For this review, take the finished solid that the model builds, in its own axes (mm). Face numbers are marked on the shaded views. A direction names the side the tool comes from. Coordinates: 2 decimals unless noted, no trailing zeros. Order: outer loops, then holes, each group sorted by start corner. A loop starts at its lowest first (then second) coordinate and runs counter-clockwise, first axis right, second up. Notation, with made-up numbers: (88, -24.5) -> (125, -24.5) arc R15 ccw to (125, -1.5) -> close; hole circle Ø8 at (84.5, -37). An arc over 180 degrees is marked (long way). Write item = value, one per line. Start each with the question number.
1) Consider section C-C on z = -25. Give the boundary of the cut face in (x, y), and give its area (3 significant figures).
2) Insertion check: pin 1 Ø8 at (x, y) = (-24.5, 14) entering from +Z; pin 2 Ø1 at (y, z) = (8, -37.5) entering from +X; pin 3 Ø3 at (x, y) = (-27, 6.5) entering from -Z; pin 4 Ø3 at (x, y) = (-26, 5) entering from -Z. Each pin has a flat end and moves straight along its axis. Give the tip position at first contact, or say it passes through.
3) Wall thickness on probe 1 along Y at (x, z) = (-26, -28.7); probe 2 along X at (y, z) = (9, -33); probe 3 along Z at (x, y) = (-6, 5.5): over which ranges is each line inside the solid? List them lowest first. Write a range as [from, to].
4) Consider section A-A on x = -26. Give the boundary of the cut face in (y, z), and give its area (3 significant figures).
5) Machinability: for the marked faces 1, 2, 3 and 4, which of the approach directions +Z, -Z, +X, -X, +Y, -Y give a long, thin tool a straight path to every point of the face, cutting with its end or side? Answer none if there is none.
6) Consider section D-D on x = -6. Give the boundary of the cut face in (y, z), and give its area (3 significant figures).
7) Consider section B-B on y = 15. Give the boundary of the cut face in (x, z).
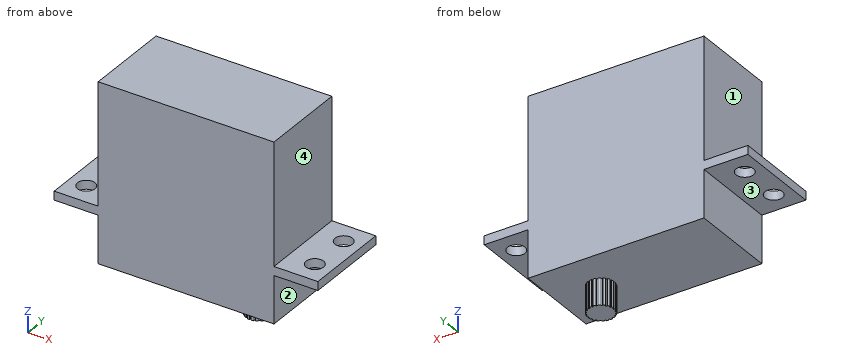
Autodesk Inventor part; units mm, degrees
ref_plane "YZ Plane" through (0, 0, 0) normal (1, 0, 0) x (0, 1, 0)
ref_plane "XZ Plane" through (0, 0, 0) normal (0, 1, 0) x (-1, 0, 0)
ref_plane "XY Plane" through (0, 0, 0) normal (0, 0, 1) x (1, 0, 0)
sketch "Sketch1" plane through (0, 0, 0) normal (0, 1, 0) x (-1, 0, 0)
  line L0 (-20, 0) -> (20, 0)
  line L1 (20, 0) -> (20, -40.5)
  line L2 (20, -40.5) -> (-20, -40.5)
  line L3 (-20, -40.5) -> (-20, 0)
  point P0 (0, 0)
  point P1 (0, -40.5)
  dimension "d0" = 40
  dimension "d1" = 40.5
extrude "Extrusion1" add sketch "Sketch1" along normal blind 20
sketch "Sketch2" plane through (20, 0, 0) normal (1, 0, 0) x (0, 0, -1)
  line L0 (27.7, 20) -> (29.7, 20)
  line L1 (29.7, 20) -> (29.7, 0)
  line L2 (29.7, 0) -> (27.7, 0)
  line L3 (27.7, 0) -> (27.7, 20)
  line L4 (40.5, 0) -> (40.5, 20)
  line L5 (0, 0) -> (0, 20)
  dimension "d4" = 2
  dimension "d31" = 27.7
extrude "Extrusion2" add sketch "Sketch2" along normal blind 10
sketch "Sketch3" plane through (20, 0, -29.7) normal (0, 0, -1) x (-1, 0, 0)
  circle A0 centre (-6, 15) radius 2
  line L0 (-10, 20) -> (-10, 0)
  line L1 (-10, 10) -> (0, 10)
  circle A1 centre (-6, 5) radius 2
  point P0 (20, 0)
  point P1 (-10, 5)
  point P2 (-8, 3.2679)
  dimension "d9" = 4
  dimension "d13" = 5
  dimension "d32" = 4
extrude "Extrusion3" cut sketch "Sketch3" against normal up to next
sketch "Sketch4" plane through (20, 0, -40.5) normal (0, 0, -1) x (-1, 0, 0)
  circle A0 centre (10, 10) radius 3
  line L0 (0, 0) -> (0, 20)
  line L1 (0, 20) -> (40, 20)
  point P0 (20, 0)
  dimension "d16" = 6
  dimension "d17" = 10
  dimension "d18" = 10
extrude "Extrusion4" add sketch "Sketch4" along normal blind 6
sketch "Sketch5" plane through (10, 10, -46.5) normal (0, 0, -1) x (-1, 0, 0)
  circle A0 centre (0, 0) radius 3
  line L0 (2.75, -0.1872) -> (3.25, -0.1872)
  line L1 (3.25, -0.1872) -> (3.25, 0.1872)
  line L2 (3.25, 0.1872) -> (2.75, 0.1872)
  line L3 (2.75, 0.1872) -> (2.75, -0.1872)
  line L4 (2.75, -0.1872) -> (3.25, 0.1872) construction
  line L5 (3.25, -0.1872) -> (2.75, 0.1872) construction
  line L6 (2.5575, 1.0279) -> (2.6733, 0.6717)
  line L7 (3.0331, 1.1824) -> (2.5575, 1.0279)
  line L8 (3.1488, 0.8262) -> (3.0331, 1.1824)
  line L9 (2.6733, 0.6717) -> (3.1488, 0.8262)
  line L10 (2.1147, 1.7679) -> (2.3348, 1.4649)
  line L11 (2.5193, 2.0618) -> (2.1147, 1.7679)
  line L12 (2.7394, 1.7588) -> (2.5193, 2.0618)
  line L13 (2.3348, 1.4649) -> (2.7394, 1.7588)
  line L14 (1.4649, 2.3348) -> (1.7679, 2.1147)
  line L15 (1.7588, 2.7394) -> (1.4649, 2.3348)
  line L16 (2.0618, 2.5193) -> (1.7588, 2.7394)
  line L17 (1.7679, 2.1147) -> (2.0618, 2.5193)
  line L18 (0.6717, 2.6733) -> (1.0279, 2.5575)
  line L19 (0.8262, 3.1488) -> (0.6717, 2.6733)
  line L20 (1.1824, 3.0331) -> (0.8262, 3.1488)
  line L21 (1.0279, 2.5575) -> (1.1824, 3.0331)
  line L22 (-0.1872, 2.75) -> (0.1872, 2.75)
  line L23 (-0.1872, 3.25) -> (-0.1872, 2.75)
  line L24 (0.1872, 3.25) -> (-0.1872, 3.25)
  line L25 (0.1872, 2.75) -> (0.1872, 3.25)
  line L26 (-1.0279, 2.5575) -> (-0.6717, 2.6733)
  line L27 (-1.1824, 3.0331) -> (-1.0279, 2.5575)
  line L28 (-0.8262, 3.1488) -> (-1.1824, 3.0331)
  line L29 (-0.6717, 2.6733) -> (-0.8262, 3.1488)
  line L30 (-1.7679, 2.1147) -> (-1.4649, 2.3348)
  line L31 (-2.0618, 2.5193) -> (-1.7679, 2.1147)
  line L32 (-1.7588, 2.7394) -> (-2.0618, 2.5193)
  line L33 (-1.4649, 2.3348) -> (-1.7588, 2.7394)
  line L34 (-2.3348, 1.4649) -> (-2.1147, 1.7679)
  line L35 (-2.7394, 1.7588) -> (-2.3348, 1.4649)
  line L36 (-2.5193, 2.0618) -> (-2.7394, 1.7588)
  line L37 (-2.1147, 1.7679) -> (-2.5193, 2.0618)
  line L38 (-2.6733, 0.6717) -> (-2.5575, 1.0279)
  line L39 (-3.1488, 0.8262) -> (-2.6733, 0.6717)
  line L40 (-3.0331, 1.1824) -> (-3.1488, 0.8262)
  line L41 (-2.5575, 1.0279) -> (-3.0331, 1.1824)
  line L42 (-2.75, -0.1872) -> (-2.75, 0.1872)
  line L43 (-3.25, -0.1872) -> (-2.75, -0.1872)
  line L44 (-3.25, 0.1872) -> (-3.25, -0.1872)
  line L45 (-2.75, 0.1872) -> (-3.25, 0.1872)
  line L46 (-2.5575, -1.0279) -> (-2.6733, -0.6717)
  line L47 (-3.0331, -1.1824) -> (-2.5575, -1.0279)
  line L48 (-3.1488, -0.8262) -> (-3.0331, -1.1824)
  line L49 (-2.6733, -0.6717) -> (-3.1488, -0.8262)
  line L50 (-2.1147, -1.7679) -> (-2.3348, -1.4649)
  line L51 (-2.5193, -2.0618) -> (-2.1147, -1.7679)
  line L52 (-2.7394, -1.7588) -> (-2.5193, -2.0618)
  line L53 (-2.3348, -1.4649) -> (-2.7394, -1.7588)
  line L54 (-1.4649, -2.3348) -> (-1.7679, -2.1147)
  line L55 (-1.7588, -2.7394) -> (-1.4649, -2.3348)
  line L56 (-2.0618, -2.5193) -> (-1.7588, -2.7394)
  line L57 (-1.7679, -2.1147) -> (-2.0618, -2.5193)
  line L58 (-0.6717, -2.6733) -> (-1.0279, -2.5575)
  line L59 (-0.8262, -3.1488) -> (-0.6717, -2.6733)
  line L60 (-1.1824, -3.0331) -> (-0.8262, -3.1488)
  line L61 (-1.0279, -2.5575) -> (-1.1824, -3.0331)
  line L62 (0.1872, -2.75) -> (-0.1872, -2.75)
  line L63 (0.1872, -3.25) -> (0.1872, -2.75)
  line L64 (-0.1872, -3.25) -> (0.1872, -3.25)
  line L65 (-0.1872, -2.75) -> (-0.1872, -3.25)
  line L66 (1.0279, -2.5575) -> (0.6717, -2.6733)
  line L67 (1.1824, -3.0331) -> (1.0279, -2.5575)
  line L68 (0.8262, -3.1488) -> (1.1824, -3.0331)
  line L69 (0.6717, -2.6733) -> (0.8262, -3.1488)
  line L70 (1.7679, -2.1147) -> (1.4649, -2.3348)
  line L71 (2.0618, -2.5193) -> (1.7679, -2.1147)
  line L72 (1.7588, -2.7394) -> (2.0618, -2.5193)
  line L73 (1.4649, -2.3348) -> (1.7588, -2.7394)
  line L74 (2.3348, -1.4649) -> (2.1147, -1.7679)
  line L75 (2.7394, -1.7588) -> (2.3348, -1.4649)
  line L76 (2.5193, -2.0618) -> (2.7394, -1.7588)
  line L77 (2.1147, -1.7679) -> (2.5193, -2.0618)
  line L78 (2.6733, -0.6717) -> (2.5575, -1.0279)
  line L79 (3.1488, -0.8262) -> (2.6733, -0.6717)
  line L80 (3.0331, -1.1824) -> (3.1488, -0.8262)
  line L81 (2.5575, -1.0279) -> (3.0331, -1.1824)
  point P0 (10, -10)
  point P1 (3, 0)
  dimension "d21" = 0.5
  dimension "d24" = 360
extrude "Extrusion5" cut sketch "Sketch5" against normal up to surface (6 mm away) contours A0 L0 L3 L2 | A0 L2 L1 L0
pattern_circular "Circular Pattern1" count 20 over 360 about axis through (10, 10, -46.5) along (0, 0, -1) of "Extrusion5"
mirror "Mirror1" about plane through (0, 0, 0) normal (1, 0, 0) of "Extrusion2", "Extrusion3"
properties part number "Servo" material "PLA"
Answer sheet:
q1.outline = (-20, 0) -> (20, 0) -> (20, 20) -> (-20, 20) -> close
q1.area = 800 mm2
q2.pin_1 = -27.7
q2.pin_2 = 20
q2.pin_3 = -29.7
q2.pin_4 = through
q3.probe_1 = [0, 3], [7, 13], [17, 20]
q3.probe_2 = [-20, 20]
q3.probe_3 = [-40.5, 0]
q4.outline = (0, -29.7) -> (3, -29.7) -> (3, -27.7) -> (0, -27.7) -> close; (7, -29.7) -> (13, -29.7) -> (13, -27.7) -> (7, -27.7) -> close; (17, -29.7) -> (20, -29.7) -> (20, -27.7) -> (17, -27.7) -> close
q4.area = 24.0 mm2
q5.face_1 = +Z, -X, +Y, -Y
q5.face_2 = -Z, +X, +Y, -Y
q5.face_3 = -Z, -X, +Y, -Y
q5.face_4 = +Z, +X, +Y, -Y
q6.outline = (0, -40.5) -> (20, -40.5) -> (20, 0) -> (0, 0) -> close
q6.area = 810 mm2
q7.outline = (-30, -29.7) -> (-28, -29.7) -> (-28, -27.7) -> (-30, -27.7) -> close; (-24, -29.7) -> (-20, -29.7) -> (-20, -40.5) -> (20, -40.5) -> (20, -29.7) -> (24, -29.7) -> (24, -27.7) -> (20, -27.7) -> (20, 0) -> (-20, 0) -> (-20, -27.7) -> (-24, -27.7) -> close; (28, -29.7) -> (30, -29.7) -> (30, -27.7) -> (28, -27.7) -> close
